```python
from build123d import *

# Parameters (mm, degrees)
COVER_FEATURE11_13X8_8_R0_6_H1_5_DEPTH    = 3
SKETCH_5_R                                = 0.75
LOCATING_PINS_D1_5_PITCH8_LENGTH1_8_DEPTH = 1.8
CHAMFER_1_SIZE                            = 0.5


with BuildPart() as part:
    # 草图4 → Cover_feature11_13x8.8_R0.6_H1.5 (new body)
    with BuildSketch(Plane.XY):
        with BuildLine():
            Line((-5.9, -4.4), (5.9, -4.4))
            ThreePointArc((5.9, -4.4), (6.324264069, -4.224264069), (6.5, -3.8))
            Line((6.5, -3.8), (6.5, 3.8))
            ThreePointArc((6.5, 3.8), (6.324264069, 4.224264069), (5.9, 4.4))
            Line((5.9, 4.4), (-5.9, 4.4))
            ThreePointArc((-5.9, 4.4), (-6.324264069, 4.224264069), (-6.5, 3.8))
            Line((-6.5, 3.8), (-6.5, -3.8))
            ThreePointArc((-6.5, -3.8), (-6.324264069, -4.224264069), (-5.9, -4.4))
        make_face()
    extrude(amount=COVER_FEATURE11_13X8_8_R0_6_H1_5_DEPTH)

    # 草图5 → Locating_pins_D1.5_pitch8_length1.8 (add)
    with BuildSketch(Plane.XY):
        with Locations((-4, 0)):
            Circle(SKETCH_5_R)
        with Locations((4, 0)):
            Circle(SKETCH_5_R)
    extrude(amount=-LOCATING_PINS_D1_5_PITCH8_LENGTH1_8_DEPTH)

    # 倒角1
    chamfer_1_edges = [part.edges().sort_by_distance(p)[0] for p in [
        (6.324264069, -4.224264069, 3),
        (6.5, 0, 3),
        (6.324264069, 4.224264069, 3),
        (0, 4.4, 3),
        (-6.324264069, 4.224264069, 3),
        (-6.5, 0, 3),
        (-6.324264069, -4.224264069, 3),
        (0, -4.4, 3),
    ]]
    chamfer(chamfer_1_edges, length=CHAMFER_1_SIZE)


solid = part.part
```
The listing builds one solid part. Answer for the finished solid, in the listing's coordinates (mm). A direction names the side the tool comes from. Coordinates: 2 decimals unless noted, no trailing zeros. Write each loop counter-clockwise with the first axis right and the second up, starting at its lowest first coordinate (ties: lowest second). Pieces come first, ordered by that corner, then holes. Notation, with made-up numbers: (1.5, -20.5) - (26.5, -20.5) arc R18 cw to (26.5, 8.5) - close; hole circle Ø10 at (65.25, 18.5). An arc over 180 degrees is marked (long way). Return JSON: item names as keys, results as strings. Group by question number.
Q1. A flat-ended cylindrical pin translates along its axis: pin 1 Ø5 at (x, y) = (0, -2.5) entering from -Z. Find the tip coordinate at first contact, or state that the pin passes through.
Q2. The part is cut by section D-D on y = 0. Write down the section's boundary in (x, z).
Q3. For a pull along X with two mould halves and no side action, classify faces 1 (the flat face through (-6.5, 0, 1)), 2 (the flat face through (4, 0, -1.8)), 3 (the cylindrical face through (-4.75, 0.03, -0.89)) as +X half, -X half, draft (parallel to the pull), parting line (faces both ways), or undercut.
Q4. The part is cut by section C-C on y = 1.25. Write down the section's boundary in (x, z).
Q5. The part is cut by section A-A on x = -4. Write down the section's boundary in (y, z).
Q6. Which of the six approach directions +Z, -Z, +X, -X, +Y, -Y give full straight-line access (tool end or side, diameter ignored) to faces 4 (the cylindrical face through (3.25, 0.03, -0.89)), 5 (the flat face through (-4, 0, -1.8))?
Q7. Find the intervals of material crossed by line 1 along Z through (x, y) = (-4.75, 1.5); line 2 along Z through (x, y) = (5.25, 4); line 3 along X through (y, z) = (3.5, 2.7), in increasing order. Write a range as [from, to].
Q8. The part is cut by section B-B on z = -0.85. Write down the section's boundary in (x, y).
Evaluation:
{
 "1": {"pin 1": "stops at z = 0"},
 "2": {"outline": "(-6.5, 0) - (-4.75, 0) - (-4.75, -1.8) - (-3.25, -1.8) - (-3.25, 0) - (3.25, 0) - (3.25, -1.8) - (4.75, -1.8) - (4.75, 0) - (6.5, 0) - (6.5, 2.5) - (6, 3) - (-6, 3) - (-6.5, 2.5) - close"},
 "3": {"face 1": "-X half", "face 2": "draft", "face 3": "undercut"},
 "4": {"outline": "(-6.5, 0) - (6.5, 0) - (6.5, 2.5) - (6, 3) - (-6, 3) - (-6.5, 2.5) - close"},
 "5": {"outline": "(-4.4, 0) - (-0.75, 0) - (-0.75, -1.8) - (0.75, -1.8) - (0.75, 0) - (4.4, 0) - (4.4, 2.5) - (3.9, 3) - (-3.9, 3) - (-4.4, 2.5) - close"},
 "6": {"face 4": "-Z", "face 5": "-Z, +X, -X, +Y, -Y"},
 "7": {"line 1": "z = [0, 3]", "line 2": "z = [0, 2.9]", "line 3": "x = [-6.3, 6.3]"},
 "8": {"outline": "circle Ø1.5 at (-4, 0); circle Ø1.5 at (4, 0)"}
}
